```python
from build123d import *

# Parameters (mm, degrees)
F1_DEPTH = 6


with BuildPart() as f1:
    # F0 (on Front) → F1 (new body)
    with BuildSketch(Plane.XZ):
        with BuildLine():
            ThreePointArc((8.998838, -0.144643), (0, -9), (-8.998838, -0.144643))
            ThreePointArc((-8.998838, -0.144643), (-9, 0), (-8.998838, 0.144643))
            Line((-8.998838, 0.144643), (-8.998838, 19.865004))
            ThreePointArc((-8.998838, 19.865004), (-19.511425, 19.364835), (-30, 18.496231))
            Line((-30, 18.496231), (-30, -50))
            ThreePointArc((-30, -50), (0, -20), (30, -50))
            Line((30, -50), (30, 18.496231))
            ThreePointArc((30, 18.496231), (19.511425, 19.364835), (8.998838, 19.865004))
            Line((8.998838, 19.865004), (8.998838, 0.144643))
            ThreePointArc((8.998838, 0.144643), (8.999709, 0.072324), (9, 0))
            ThreePointArc((9, 0), (8.999709, -0.072324), (8.998838, -0.144643))
        make_face()
        with BuildLine():
            ThreePointArc((30, -50), (0, -20), (-30, -50))
            ThreePointArc((-30, -50), (0, -80), (30, -50))
        make_face()
    extrude(amount=F1_DEPTH)


solid = f1.part
```
Geometry check sheet. Reference: the model listing, model coordinates, mm. A direction names the side the tool comes from. Give positions to 0.01 mm unless a question says otherwise; leave off trailing zeros. Loops run counter-clockwise (first coordinate to the right, second up) from the corner with the lowest first, then second, coordinate; pieces in that order, holes last. Notation, with made-up numbers: (26.5, 59) - (76.5, 59) arc R12 cw to (76.5, 65) - close; hole circle Ø4 at (-22.5, 78.5). An arc over 180 degrees is marked (long way). Use CSV: the item, a comma, the result in double quotes. Start each with the question number.
Q1. Scan lines: probe 1 along X at (y, z) = (-1.6, -5); probe 2 along X at (y, z) = (-2.8, -4); probe 3 along X at (y, z) = (-5.65, -60). Record each from-to range of solid material in increasing order. Write a range as from..to.
Q2. Release check for a two-part mould opening along Z. For faces 3 (the face through (19.658, -2.958, 19.355)), 4 (the face through (8.999, -3, 10)), 5 (the face through (-0.66, -2.958, -79.993)) record: +Z half, -Z half, draft (parallel to the pull), parting line (faces both ways), or undercut.
Q3. Section check B-B, the plane y = -2.15. Record the cut outline in (x, z) (3 decimals), and give its area (3 significant figures).
Q4. Access from +Z, -Z, +X, -X, +Y, -Y to the whole of each face (thin tool, end or side, straight path). Record for faces 1 (the face through (0, 0, -29)), 2 (the face through (-8.999, -3, 10)).
Q5. Section check D-D, the plane z = -61. Record the cut outline in (x, y), and give its area (3 significant figures).
Q6. Section check C-C, the plane x = 0. Record the cut outline in (y, z).
Q7. Go/stop test with flat-tipped pins: pin 1 Ø2 at (y, z) = (-3, -66.5) entering from -X; pin 2 Ø2 at (y, z) = (-3.5, -58.5) entering from +X; pin 3 Ø1.5 at (x, y) = (1, -4) entering from -Z. Record where each tip stops, or that it passes through.
Q8. Section check A-A, the plane z = 12. Record the cut outline in (x, y), and give its area (3 significant figures).
Findings below:
1,probe 1,"x = -30..-7.48, 7.48..30"
1,probe 2,"x = -30..-8.06, 8.06..30"
1,probe 3,"x = -28.28..28.28"
2,face 3,"+Z half"
2,face 4,"draft"
2,face 5,"-Z half"
3,outline,"(-30, -50) arc R30 ccw to (30, -50) - (30, 18.496) arc R299.999 ccw to (8.999, 19.865) - (8.999, 0.145) arc R9.018 cw to (9, 0) arc R9.018 cw to (8.999, -0.145) arc R9 cw to (-8.999, -0.145) arc R9.003 cw to (-8.999, 0.145) - (-8.999, 19.865) arc R299.999 ccw to (-30, 18.496) - close"
3,area,"5,100 mm^2"
4,face 1,"+Z, -Z, +X, -X, +Y"
4,face 2,"+Z, +Y, -Y"
5,outline,"(-27.91, -6) - (27.91, -6) - (27.91, 0) - (-27.91, 0) - close"
5,area,"335 mm^2"
6,outline,"(-6, -80) - (0, -80) - (0, -9) - (-6, -9) - close"
7,pin 1,"stops at x = -25.69"
7,pin 2,"stops at x = 29.05"
7,pin 3,"stops at z = -80"
8,outline,"(-30, -6) - (-9, -6) - (-9, 0) - (-30, 0) - close; (9, -6) - (30, -6) - (30, 0) - (9, 0) - close"
8,area,"252 mm^2"
